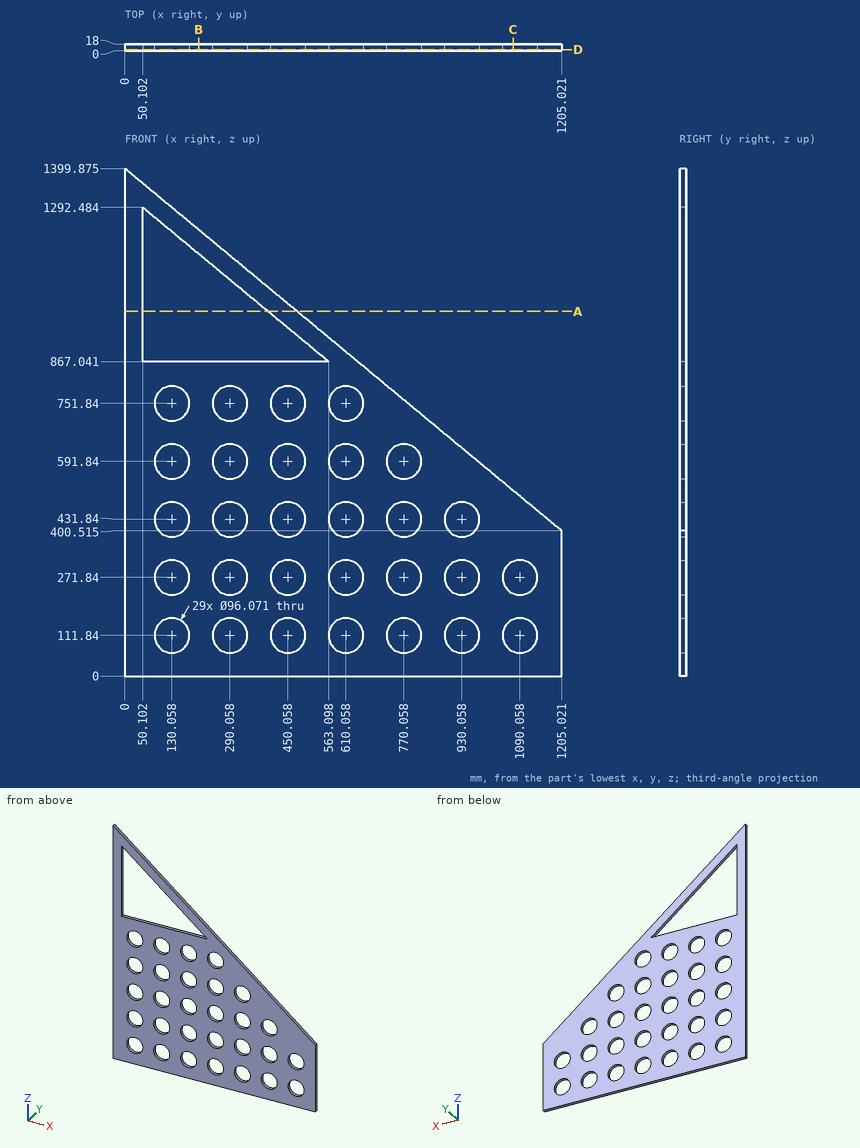
Source: three-view drawing plus pictorial views. Frame: mm from the lowest corner of the part. Coordinates: 2 decimals unless noted, no trailing zeros. Loops run counter-clockwise (first coordinate to the right, second up) from the corner with the lowest first, then second, coordinate; pieces in that order, holes last. Notation, with made-up numbers: M 65.25,85.5 L 117.25,85.5 A20 cw 117.25,122.5 Z; hole C 4.5,38 d3. An arc over 180 degrees is marked long. Use CSV: the item, a comma, the result in double quotes.
(1) Line query: line 1 (Z direction, x = 973.5, y = 10.5) (1 decimal); line 2 (X direction, y = 3.25, z = 787) (1 decimal); line 3 (Z direction, x = 907, y = 9.75) (1 decimal). Output: solid intervals per line, ascending. Write a range as [from, to].
Answers follow:
line 1,"[0, 91.3], [132.3, 251.3], [292.3, 411.3], [452.3, 592.5]"
line 2,"[0, 97.3], [162.8, 257.3], [322.8, 417.3], [482.8, 577.3], [642.8, 739]"
line 3,"[0, 69.7], [154, 229.7], [314, 389.7], [474, 647.7]"
(2) Contact query for flat-ended pins moving along their axis: pin 1 (1.5 mm diameter, centred on x = 819.5, y = 6.5, fed in from +Z); pin 2 (6 mm diameter, centred on x = 692.5, y = 11.5, fed in from +Z). Output: stop coordinate, or through.
Answers follow:
pin 1,"z = 720.86"
pin 2,"z = 828.05"
(3) Cut plane B-B on x = 203.5. Return loops of the section in (y, z), and give its area (3 significant figures).
Answers follow:
outline,"M 0,0 L 18,0 L 18,867.04 L 0,867.04 Z; M 0,1165.27 L 18,1165.27 L 18,1231.11 L 0,1231.11 Z"
area,"16,800 mm²"
(4) Cut plane A-A on z = 1005.5. Return loops of the section in (x, y) (1 decimal).
Answers follow:
outline,"M 0,0 L 50.1,0 L 50.1,18 L 0,18 Z; M 396.1,0 L 475.5,0 L 475.5,18 L 396.1,18 Z"
(5) Cut plane D-D on y = 2.75. Give the number of separate pieces and of enclosed holes in the cut face, and give its area (3 significant figures).
Answers follow:
separate pieces,"1"
enclosed holes,"30"
area,"765,000 mm²"
(6) Cut plane C-C on x = 1071. Return loops of the section in (y, z).
Answers follow:
outline,"M 0,0 L 18,0 L 18,67.75 L 0,67.75 Z; M 0,155.93 L 18,155.93 L 18,227.75 L 0,227.75 Z; M 0,315.93 L 18,315.93 L 18,511.66 L 0,511.66 Z"
